Model file for the job. Use its own axes, mm. Face numbers are marked on the shaded views. A direction names the side the tool comes from. Give positions to 0.01 mm unless a question says otherwise; leave off trailing zeros. Order: outer loops, then holes, each group sorted by start corner. A loop starts at its lowest first (then second) coordinate and runs counter-clockwise, first axis right, second up. Notation, with made-up numbers: (54.5, -26.5) -> (111.5, -26.5) arc R5 cw to (111.5, -18.5) -> close; hole circle Ø9 at (41.25, -29.5). An arc over 180 degrees is marked (long way). Use CSV: the item, a comma, the result in double quotes. Start each with the question number.
1. Cut at B-B on x = -67.31. List the corners of the cut face in (y, z), then the cut area to 3 significant figures.
2. Cut at A-A on x = -38.5. List the corners of the cut face in (y, z).
3. Drop flat-ended pins along their axis: pin 1 (12.5 mm diameter, centred on y = 0, z = 35.052, fed in from +X); pin 2 (12 mm diameter, centred on x = 15, z = 3, fed in from -Y); pin 3 (13 mm diameter, centred on y = 0.5, z = -0.5, fed in from -X); pin 4 (1 mm diameter, centred on y = 10, z = 10.5, fed in from -X). Give the stop position or say it passes through.
4. Wall check: line 1 (X direction, y = 16, z = 4.5); line 2 (Z direction, x = 16, y = 4); line 3 (Z direction, x = -67.31, y = 6.6). Give the ranges that are in metal, low to high. Write a range as from..to.
5. 3-axis set-ups, long thin cutter, end or side, ignore diameter. For the marked faces 1, 2 and 3: which of +Z, -Z, +X, -X, +Y, -Y reach the whole face in a straight line?
```python
from build123d import *

# Parameters (mm, degrees)
HOLE1_D            = 7.874
HOLE1_DEPTH        = 7.62
SKETCH5_R          = 3.937
CUT_EXTRUDE5_DEPTH = 43.688


with BuildPart() as part:
    # Sketch2 → Revolve1 (revolve)
    with BuildSketch(Plane.XY, mode=Mode.PRIVATE) as revolve1_sk:
        Polygon((-78.74, 8.001), (-78.74, 5.901826446), (-53.34, 5.901826446), (-53.34, 0), (53.34, 0), (53.34, 8.001), (43.688, 8.001), (43.688, 44.069), (40.386, 44.069), (40.386, 8.001), align=None)
    revolve(revolve1_sk.sketch.rotate(Axis((-53.34, 0, 0), (1, 0, 0)), 180), axis=Axis((-53.34, 0, 0), (1, 0, 0)))

    # Hole1
    with Locations(Plane(origin=(-67.31, 8.001, 0), x_dir=(0, 0, 1), z_dir=(0, 1, 0))):
        with Locations((0, 0)):
            Hole(HOLE1_D / 2, depth=HOLE1_DEPTH)

    # Sketch5 → Cut-Extrude5 (cut)
    with BuildSketch(Plane(origin=(0, 0, 0), x_dir=(0, 0, -1), z_dir=(1, 0, 0))):
        with BuildLine():
            ThreePointArc((-8.064098995, 39.086426403), (-4.739613176, 42.72287713), (0, 44.069))
            ThreePointArc((0, 44.069), (-31.16148874, 31.16148874), (-44.069, 0))
            ThreePointArc((-44.069, 0), (-42.72287713, 4.739613176), (-39.086426403, 8.064098995))
            add(Edge.make_bspline(
                [(-39.086426403, 8.064098995), (-32.863680484, 12.182521195), (-14.294768831, 14.295822644), (-12.182274492, 32.864426866), (-8.064098995, 39.086426403)],
                knots=[0, 0, 0, 0, 0.500028123, 1, 1, 1, 1], degree=3))
        make_face()
        with BuildLine():
            ThreePointArc((-44.069, 0), (-31.16148874, -31.16148874), (0, -44.069))
            ThreePointArc((0, -44.069), (-4.739613176, -42.72287713), (-8.064098995, -39.086426403))
            add(Edge.make_bspline(
                [(-8.064098995, -39.086426403), (-12.182485102, -32.863323284), (-14.296876524, -14.294960375), (-32.864680523, -12.182036473), (-39.086426403, -8.064098995)],
                knots=[0, 0, 0, 0, 0.50005114, 1, 1, 1, 1], degree=3))
            ThreePointArc((-39.086426403, -8.064098995), (-42.72287713, -4.739613176), (-44.069, 0))
        make_face()
        with Locations(Location((0, -35.052, 0), (0, 0, 270))):
            Circle(SKETCH5_R)
        with BuildLine():
            ThreePointArc((0, -44.069), (31.16148874, -31.16148874), (44.069, 0))
            ThreePointArc((44.069, 0), (42.72287713, -4.739613176), (39.086426403, -8.064098995))
            add(Edge.make_bspline(
                [(39.086426403, -8.064098995), (32.863323284, -12.182485102), (14.294960375, -14.296876524), (12.182036473, -32.864680523), (8.064098995, -39.086426403)],
                knots=[0, 0, 0, 0, 0.50005114, 1, 1, 1, 1], degree=3))
            ThreePointArc((8.064098995, -39.086426403), (4.739613176, -42.72287713), (0, -44.069))
        make_face()
        with Locations(Location((35.052, 0, 0), (0, 0, 270))):
            Circle(SKETCH5_R)
        with BuildLine():
            ThreePointArc((39.086426403, 8.064098995), (42.72287713, 4.739613176), (44.069, 0))
            ThreePointArc((44.069, 0), (31.16148874, 31.16148874), (0, 44.069))
            ThreePointArc((0, 44.069), (4.739613176, 42.72287713), (8.064098995, 39.086426403))
            add(Edge.make_bspline(
                [(8.064098995, 39.086426403), (12.182485102, 32.863323284), (14.296876524, 14.294960375), (32.864680523, 12.182036473), (39.086426403, 8.064098995)],
                knots=[0, 0, 0, 0, 0.50005114, 1, 1, 1, 1], degree=3))
        make_face()
        with Locations(Location((0, 35.052, 0), (0, 0, 270))):
            Circle(SKETCH5_R)
        with Locations(Location((-35.052, 0, 0), (0, 0, 270))):
            Circle(SKETCH5_R)
    extrude(amount=CUT_EXTRUDE5_DEPTH, mode=Mode.SUBTRACT)


solid = part.part
```
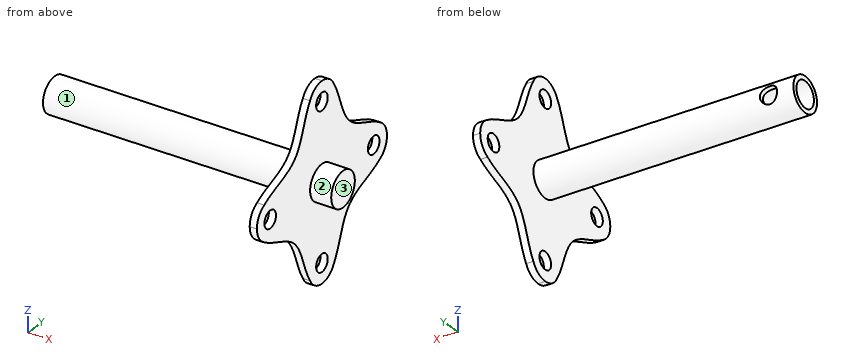
Verdict:
1,outline,"(4.4, -3.94) arc R5.9 cw (long way) to (4.4, 3.94) -> (6.97, 3.94) arc R8 ccw (long way) to (6.97, -3.94) -> close"
1,area,"74.1 mm^2"
2,outline,"circle Ø16 at (0, 0)"
3,pin 1,"x = 43.69"
3,pin 2,"y = -8"
3,pin 3,"x = -78.74"
3,pin 4,"x = 40.39"
4,line 1,"40.39..43.69"
4,line 2,"-6.93..6.93"
4,line 3,"-4.52..-3.94, 3.94..4.52"
5,face 1,"-X"
5,face 2,"+X"
5,face 3,"+Z, -Z, +X, +Y, -Y"
